from build123d import *

# Parameters (mm, degrees)
F0_R     = 15
F1_DEPTH = 400
F2_R     = 10
F3_DEPTH = 10
F4_R     = 0.5
F5_SIZE  = 1
F6_W     = 1
F6_H     = 2


with BuildPart() as f1:
    # F0 (on Top) → F1 (new body)
    with BuildSketch(Plane.XY):
        Circle(F0_R)
    extrude(amount=-F1_DEPTH)

    # F2 (on face) → F3 (join)
    with BuildSketch(Plane.XY):
        Circle(F2_R)
    extrude(amount=F3_DEPTH)

    # F4
    f4_edges = [f1.edges().sort_by_distance(p)[0] for p in [
        (-15, 0, -400),
        (-15, 0, 0),
    ]]
    fillet(f4_edges, radius=F4_R)

    # F5
    f5_edges = [f1.edges().sort_by_distance(p)[0] for p in [
        (-10, 0, 10),
    ]]
    chamfer(f5_edges, length=F5_SIZE)

    # F6 (on Front) → F7 (revolve, cut)
    with BuildSketch(Plane.XZ):
        with Locations((-9.5, 1)):
            Rectangle(F6_W, F6_H)
    revolve(axis=Axis((0, 0, 12.057068), (0, 0, 1)), mode=Mode.SUBTRACT)


solid = f1.part
The model under review builds one solid part; all positions refer to its coordinate system, in mm. A direction names the side the tool comes from. Coordinates: 2 decimals unless noted, no trailing zeros. Order: outer loops, then holes, each group sorted by start corner. A loop starts at its lowest first (then second) coordinate and runs counter-clockwise, first axis right, second up. Notation, with made-up numbers: (15.5, 63) -> (23.5, 63) arc R20 ccw to (23.5, 87) -> close; hole circle Ø1 at (86.25, 82.5). An arc over 180 degrees is marked (long way). Answer in a Markdown table with one row per item.
(1) Wall thickness on line 1 along Y through (x, z) = (-0.5, -24); line 2 along Z through (x, y) = (7, -7.5); line 3 along Y through (x, z) = (12, -344): over which ranges is each line inside the solid? List them lowest first.
Answers:
| item | result |
|---|---|
| line 1 | -14.99 to 14.99 |
| line 2 | -400 to 0 |
| line 3 | -9 to 9 |
(2) Consider section A-A (z = -22.5). Write out the cut boundary in (x, y).
Answers:
| item | result |
|---|---|
| outline | circle Ø30 at (0, 0) |
(3) The part is to be moulded in two halves that separate along Z. For faces 4 (the flat face through (9, -2, 2)), 5 (the flat face through (0, 0, 10)), 6 (the cylindrical face through (1.172, -8.923, 1.014)), 7 (the cylindrical face through (-14.985, 0.66, -197.207)), say which applies: +Z half, -Z half, draft (parallel to the pull), parting line (faces both ways), or undercut.
Answers:
| item | result |
|---|---|
| face 4 | undercut |
| face 5 | +Z half |
| face 6 | undercut |
| face 7 | draft |
(4) Machinability: for faces 1 (the flat face through (6, 7, 0)), 2 (the flat face through (0, 0, -400)), 3 (the cylindrical face through (-2.17, -9.76, 5.45)), which of the approach directions +Z, -Z, +X, -X, +Y, -Y give a long, thin tool a straight path to every point of the face, cutting with its end or side? Answer none if there is none.
Answers:
| item | result |
|---|---|
| face 1 | none |
| face 2 | -Z, +X, -X, +Y, -Y |
| face 3 | +Z |
(5) Insertion check: pin 1 (8 mm diameter, centred on y = -7, z = -274, fed in from -X); pin 2 (3 mm diameter, centred on x = -8, z = -349.5, fed in from -Y); pin 3 (5 mm diameter, centred on x = 4.5, z = -357, fed in from +Y). Each pin has a flat end and moves straight along its axis. Give the tip position at first contact, or say it passes through.
Answers:
| item | result |
|---|---|
| pin 1 | x = -14.7 |
| pin 2 | y = -13.52 |
| pin 3 | y = 14.87 |
